```python
from build123d import *

# Parameters (mm, degrees)
CYLINDER012_R            = 0.9
CYLINDER012_DEPTH        = 3.5
BOX039_W                 = 5
BOX039_H                 = 5
BOX039_DEPTH             = 3.5
CLONE011_PLACEMENT_ANGLE = 45


with BuildPart() as anchorscrew:
    # Cylinder012 → Cylinder012 (new body)
    with BuildSketch(Plane(origin=(2.5, 2.5, 0), x_dir=(1, 0, 0), z_dir=(0, 0, 1))):
        Circle(CYLINDER012_R)
    extrude(amount=CYLINDER012_DEPTH)


with BuildPart() as anchor006:
    # Box039 → Box039 (new body)
    with BuildSketch(Plane.XY):
        with Locations((2.5, 2.5)):
            Rectangle(BOX039_W, BOX039_H)
    extrude(amount=BOX039_DEPTH)

    # Cut010: cut AnchorScrew
    add(anchorscrew.part, mode=Mode.SUBTRACT)


with BuildPart() as anchor006_1:
    # Clone011 placement: moved
    add(anchor006.part.moved(Location((98.326641456, 10.6550685808, 2))).rotate(Axis((98.326641456, 10.6550685808, 2), (0, 0, 1)), CLONE011_PLACEMENT_ANGLE))


with BuildPart() as part_mirroring010:
    # Part__Mirroring010: instance of Anchor006
    add(anchor006_1.part.mirror(Plane(origin=(0, 0, 5.5), x_dir=(0, 1, 0), z_dir=(0, 0, 1))))


solid = part_mirroring010.part
```
Input: part model. Units: mm. Frame: model coordinates. Round coordinates to 2 decimals unless told otherwise and drop trailing zeros. Loops run counter-clockwise (first coordinate to the right, second up) from the corner with the lowest first, then second, coordinate; pieces in that order, holes last.
1) Section query A-A on x = 98.5. Return the cut outline in (y, z).
Ans:
outline: (10.83, 5.5) - (13.31, 5.5) - (13.31, 9) - (10.83, 9) - close; (15.07, 5.5) - (17.55, 5.5) - (17.55, 9) - (15.07, 9) - close
2) Pull-direction query (Y, two-part tool) for faces 1 (the flat face through (100.07, 12.4, 7.27)), 2 (the cylindrical face through (99.16, 14.53, 7.27)), 3 (the flat face through (96.5, 15.9, 7.3)); classes: released by +Y, released by -Y, zero draft, split by the parting line, or undercut.
Ans:
face 1: released by -Y
face 2: undercut
face 3: released by +Y
3) Material intervals for line 1 (X direction, y = 14, z = 7.35); line 2 (X direction, y = 14.5, z = 8.6); line 3 (Y direction, x = 98.25, z = 6.35), sorted ascending.
Ans:
line 1: x = 94.98 to 97.45, 99.21 to 101.67
line 2: x = 95.1 to 97.48, 99.17 to 101.55
line 3: y = 10.73 to 13.29, 15.09 to 17.65
4) Section query D-D on x = 97. Return the cut outline in (y, z).
Ans:
outline: (11.98, 5.5) - (16.4, 5.5) - (16.4, 9) - (11.98, 9) - close
5) Section query C-C on z = 5.95. Return the cut outline in (x, y).
Ans:
outline: (94.79, 14.19) - (98.33, 10.66) - (101.86, 14.19) - (98.33, 17.73) - close; hole circle Ø1.8 at (98.33, 14.19)
6) Section query B-B on y = 13.75. Return the cut outline in (x, z), plus the area to 3 significant figures.
Ans:
outline: (95.23, 5.5) - (97.54, 5.5) - (97.54, 9) - (95.23, 9) - close; (99.11, 5.5) - (101.42, 5.5) - (101.42, 9) - (99.11, 9) - close
area: 16.2 mm2
7) Pin query (flat end, axial travel): pin 1 (2 mm diameter, centred on y = 16, z = 7.5, fed in from -X). Return the tip coordinate at first contact, or that it passes through.
Ans:
pin 1: stops at x = 95.6
